```python
from build123d import *

# Parameters (mm, degrees)
F0_W      = 304.8
F0_H      = 304.8
F1_DEPTH  = 4.2418
F2_W      = 25.527
F2_H      = 25.527
F2_W_2    = 22.987
F2_H_2    = 22.987
F3_DEPTH  = 228.6
F4_R      = 1.905
F5_DEPTH  = 165.1645
F6_W      = 25.527
F6_H      = 5.08
F7_DEPTH  = 25.4
F8_R      = 1.27
F9_DEPTH  = 5.08
F11_W     = 25.527
F11_H     = 5.08
F12_DEPTH = 25.4
F13_R     = 1.27
F14_DEPTH = 5.08
F15_R     = 1.905
F16_DEPTH = 165.1645


with BuildPart() as f1:
    # F0 (on Top) → F1 (new body)
    with BuildSketch(Plane.XY):
        Rectangle(F0_W, F0_H)
    extrude(amount=F1_DEPTH)

    # F2 (on face) → F3 (join)
    with BuildSketch(Plane.XY.offset(4.2418)):
        with Locations((139.6365, 0)):
            Rectangle(F2_W, F2_H)
        with Locations((139.6365, 0)):
            Rectangle(F2_W_2, F2_H_2, mode=Mode.SUBTRACT)
    extrude(amount=F3_DEPTH)

    # F4 (on face) → F5 (cut, through all)
    with BuildSketch(Plane.XZ.offset(12.7635)):
        with Locations((139.6365, 42.3418)):
            Circle(F4_R)
        with Locations((139.6365, 80.4418)):
            Circle(F4_R)
        with Locations((139.6365, 118.5418)):
            Circle(F4_R)
        with Locations((139.6365, 156.6418)):
            Circle(F4_R)
        with Locations((139.6365, 194.7418)):
            Circle(F4_R)
    extrude(amount=-F5_DEPTH, mode=Mode.SUBTRACT)

    # F6 (on face) → F7 (join)
    with BuildSketch(Plane.XZ.offset(12.7635)):
        with Locations((139.6365, 6.7818)):
            Rectangle(F6_W, F6_H)
    extrude(amount=F7_DEPTH)

    # F8 (on face) → F9 (cut)
    with BuildSketch(Plane.XY.offset(9.3218)):
        with Locations((139.6365, -25.4635)):
            Circle(F8_R)
    extrude(amount=-F9_DEPTH, mode=Mode.SUBTRACT)

    # F10: F1 across plane


with BuildPart() as f1_1:
    add(f1.part)
    add(f1.part.mirror(Plane.XZ))

    # F11 (on face) → F12 (join)
    with BuildSketch(Plane(origin=(126.873, 0, 0), x_dir=(0, -1, 0), z_dir=(-1, 0, 0))):
        with Locations((0, 6.7818)):
            Rectangle(F11_W, F11_H)
    extrude(amount=F12_DEPTH)

    # F13 (on face) → F14 (cut)
    with BuildSketch(Plane.XY.offset(9.3218)):
        with Locations((114.173, 0)):
            Circle(F13_R)
    extrude(amount=-F14_DEPTH, mode=Mode.SUBTRACT)

    # F15 (on face) → F16 (cut, through all)
    with BuildSketch(Plane.XZ.offset(12.7635)):
        with Locations((139.6365, 220.1418)):
            Circle(F15_R)
        with Locations((147.2565, 220.1418)):
            Circle(F15_R)
        with Locations((139.6365, 212.5218)):
            Circle(F15_R)
    extrude(amount=-F16_DEPTH, mode=Mode.SUBTRACT)


solid = f1_1.part
```
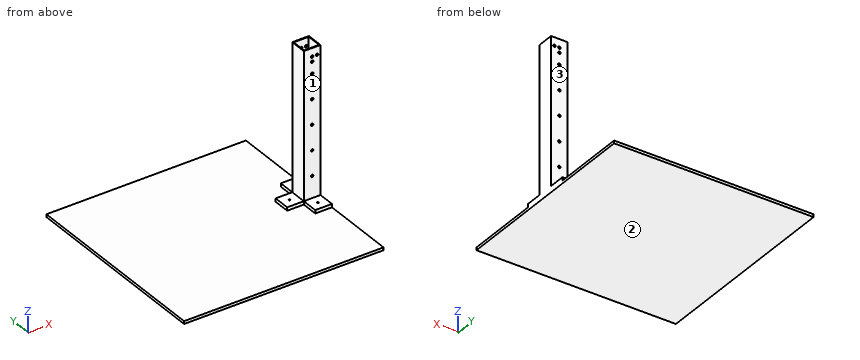
Model file for the job. Use its own axes, mm. Face numbers are marked on the shaded views. A direction names the side the tool comes from. Coordinates: 2 decimals unless noted, no trailing zeros. Order: outer loops, then holes, each group sorted by start corner. A loop starts at its lowest first (then second) coordinate and runs counter-clockwise, first axis right, second up. Notation, with made-up numbers: (-33.75, 18.25) -> (25.25, 18.25) arc R19 ccw to (25.25, 30.25) -> close; hole circle Ø9 at (53, 66). An arc over 180 degrees is marked (long way). Answer as a JSON object with one key per item and string values. Group by question number.
1) Cut at A-A, the plane z = 165.5. Write the cut outline in (x, y).
2) Flat gauge pins, fed straight in: pin 1 (4.5 mm diameter, centred on x = 139.64, z = 220.14, fed in from +Y); pin 2 (3.5 mm diameter, centred on x = 147.26, z = 220.14, fed in from +Y); pin 3 (6 mm diameter, centred on x = 94.5, y = -122, fed in from +Z); pin 4 (7.5 mm diameter, centred on x = 133.5, z = 66, fed in from -Y). Where does each tip first touch, or does it go through?
3) Which spindle directions (+Z, -Z, +X, -X, +Y, -Y) get a long thin tool onto all of the face, cutting with end or side? Do the marked faces 1, 2 and 3. Say none if no direction does.
4) Drill centre line: L1, parallel to Z at x = 37.5, y = -24.5. Where is it in solid material? Low to high.
5) Cut at B-B, the plane y = -47.5. Write the cut outline in (x, z), then the cut area to 3 significant figures.
Check values:
{
 "1": {"outline": "(126.87, -12.76) -> (152.4, -12.76) -> (152.4, 12.76) -> (126.87, 12.76) -> close; hole (128.14, -11.49) -> (151.13, -11.49) -> (151.13, 11.49) -> (128.14, 11.49) -> close"},
 "2": {"pin 1": "stops at y = 12.76", "pin 2": "passes through", "pin 3": "stops at z = 4.24", "pin 4": "stops at y = -12.76"},
 "3": {"face 1": "+Z, +X, -X, -Y", "face 2": "-Z, +X, -X, +Y, -Y", "face 3": "+Z, +X, -X, +Y"},
 "4": {"L1": "z = 0 to 4.24"},
 "5": {"outline": "(-152.4, 0) -> (152.4, 0) -> (152.4, 4.24) -> (-152.4, 4.24) -> close", "area": "1,290 mm²"}
}
